from build123d import *

# Parameters (mm, degrees)
ESBO_O1_R                = 1.6
ESBO_O1_R_2              = 1.15
RESSALTO_EXTRUS_O1_DEPTH = 2


with BuildPart() as part:
    # Esboço1 → Ressalto-extrusão1 (new body)
    with BuildSketch(Plane(origin=(0, 0, 0), x_dir=(1, 0, 0), z_dir=(0, 1, 0))):
        with BuildLine():
            Line((-47, -13), (47, -13))
            ThreePointArc((47, -13), (50.535533906, -11.535533906), (52, -8))
            Line((52, -8), (52, 8))
            ThreePointArc((52, 8), (50.535533906, 11.535533906), (47, 13))
            Line((47, 13), (-47, 13))
            ThreePointArc((-47, 13), (-50.535533906, 11.535533906), (-52, 8))
            Line((-52, 8), (-52, -8))
            ThreePointArc((-52, -8), (-50.535533906, -11.535533906), (-47, -13))
        make_face()
        with Locations((46, 8)):
            Circle(ESBO_O1_R, mode=Mode.SUBTRACT)
        with Locations((46, -8)):
            Circle(ESBO_O1_R, mode=Mode.SUBTRACT)
        with Locations((49, 0)):
            Circle(ESBO_O1_R_2, mode=Mode.SUBTRACT)
        with Locations((40, 0)):
            Circle(ESBO_O1_R_2, mode=Mode.SUBTRACT)
        with Locations((-46, 8)):
            Circle(ESBO_O1_R, mode=Mode.SUBTRACT)
        with Locations((-46, -8)):
            Circle(ESBO_O1_R, mode=Mode.SUBTRACT)
        with Locations((-40, 0)):
            Circle(ESBO_O1_R_2, mode=Mode.SUBTRACT)
        with Locations((-49, 0)):
            Circle(ESBO_O1_R_2, mode=Mode.SUBTRACT)
        with Locations((-31, 0)):
            Circle(ESBO_O1_R_2, mode=Mode.SUBTRACT)
        with BuildLine():
            Line((3.307143995, -1.544441193), (30.307143995, -1.544441193))
            Line((30.307143995, -1.544441193), (30.307143995, 1.544441193))
            Line((30.307143995, 1.544441193), (3.307143995, 1.544441193))
            ThreePointArc((3.307143995, 1.544441193), (0, 3.65), (-3.307143995, 1.544441193))
            Line((-3.307143995, 1.544441193), (-21.692856005, 1.544441193))
            Line((-21.692856005, 1.544441193), (-21.692856005, -1.544441193))
            Line((-21.692856005, -1.544441193), (-3.307143995, -1.544441193))
            ThreePointArc((-3.307143995, -1.544441193), (0, -3.65), (3.307143995, -1.544441193))
        make_face(mode=Mode.SUBTRACT)
    extrude(amount=RESSALTO_EXTRUS_O1_DEPTH)


solid = part.part
For this review, take the finished solid that the model builds, in its own axes (mm). A direction names the side the tool comes from. Coordinates: 2 decimals unless noted, no trailing zeros. Order: outer loops, then holes, each group sorted by start corner. A loop starts at its lowest first (then second) coordinate and runs counter-clockwise, first axis right, second up. Notation, with made-up numbers: (30, -4) -> (87, -4) arc R27 ccw to (87, 13) -> close; hole circle Ø4 at (74, 56.5). An arc over 180 degrees is marked (long way). Return JSON: item names as keys, results as strings.
1. We need section A-A on x = -46. Write out the cut boundary in (y, z), and give its area (3 significant figures).
Answer block:
{"outline": "(0, -13) -> (2, -13) -> (2, -9.6) -> (0, -9.6) -> close; (0, -6.4) -> (2, -6.4) -> (2, 6.4) -> (0, 6.4) -> close; (0, 9.6) -> (2, 9.6) -> (2, 13) -> (0, 13) -> close", "area": "39.2 mm²"}
2. We need section C-C on z = 0. Write out the cut boundary in (x, y), and give its area (3 significant figures).
Answer block:
{"outline": "(-52, 0) -> (-50.15, 0) -> (-50.15, 2) -> (-52, 2) -> close; (-47.85, 0) -> (-41.15, 0) -> (-41.15, 2) -> (-47.85, 2) -> close; (-38.85, 0) -> (-32.15, 0) -> (-32.15, 2) -> (-38.85, 2) -> close; (-29.85, 0) -> (-21.69, 0) -> (-21.69, 2) -> (-29.85, 2) -> close; (30.31, 0) -> (38.85, 0) -> (38.85, 2) -> (30.31, 2) -> close; (41.15, 0) -> (47.85, 0) -> (47.85, 2) -> (41.15, 2) -> close; (50.15, 0) -> (52, 0) -> (52, 2) -> (50.15, 2) -> close", "area": "81.0 mm²"}
3. We need section D-D on x = 40. Write out the cut boundary in (y, z).
Answer block:
{"outline": "(0, -13) -> (2, -13) -> (2, -1.15) -> (0, -1.15) -> close; (0, 1.15) -> (2, 1.15) -> (2, 13) -> (0, 13) -> close"}
4. The part is to be moulded in two halves that separate along Z. For faces 3 (the cylindrical face through (-0.06, 0.99, 3.65)), 4 (the flat face through (-1, 0, -6)), 5 (the cylindrical face through (50, 1, 12)), say which applies: +Z half, -Z half, draft (parallel to the pull), parting line (faces both ways), or undercut.
Answer block:
{"face 3": "undercut", "face 4": "draft", "face 5": "+Z half"}
5. For line 1 (X direction, y = 1.2, z = 8); line 2 (Z direction, x = -46, y = 0.75); line 3 (Z direction, x = 17, y = 1.85), list the stretches that pass through material, from the lowest coordinate up. Write a range as from..to.
Answer block:
{"line 1": "-52..-47.6, -44.4..44.4, 47.6..52", "line 2": "-13..-9.6, -6.4..6.4, 9.6..13", "line 3": "-13..-1.54, 1.54..13"}
6. Machinability: for faces 1 (the flat face through (-1, 2, -6)), 2 (the flat face through (-21.693, 1, 0)), which of the approach directions +Z, -Z, +X, -X, +Y, -Y give a long, thin tool a straight path to every point of the face, cutting with its end or side? Answer none if there is none.
Answer block:
{"face 1": "+Z, -Z, +X, -X, +Y", "face 2": "+Y, -Y"}
7. We need section B-B on y = 0.4. State how many separate pieces and enclosed holes the cut face has, and give its area (3 significant figures).
Answer block:
{"separate pieces": "1", "enclosed holes": "10", "area": "2,450 mm²"}
